Input: dimensioned drawing with shaded views. Units: mm. Origin: part minimum x, y, z. Give positions to 0.01 mm unless a question says otherwise; leave off trailing zeros. Write each loop counter-clockwise with the first axis right and the second up, starting at its lowest first coordinate (ties: lowest second). Pieces come first, ordered by that corner, then holes.
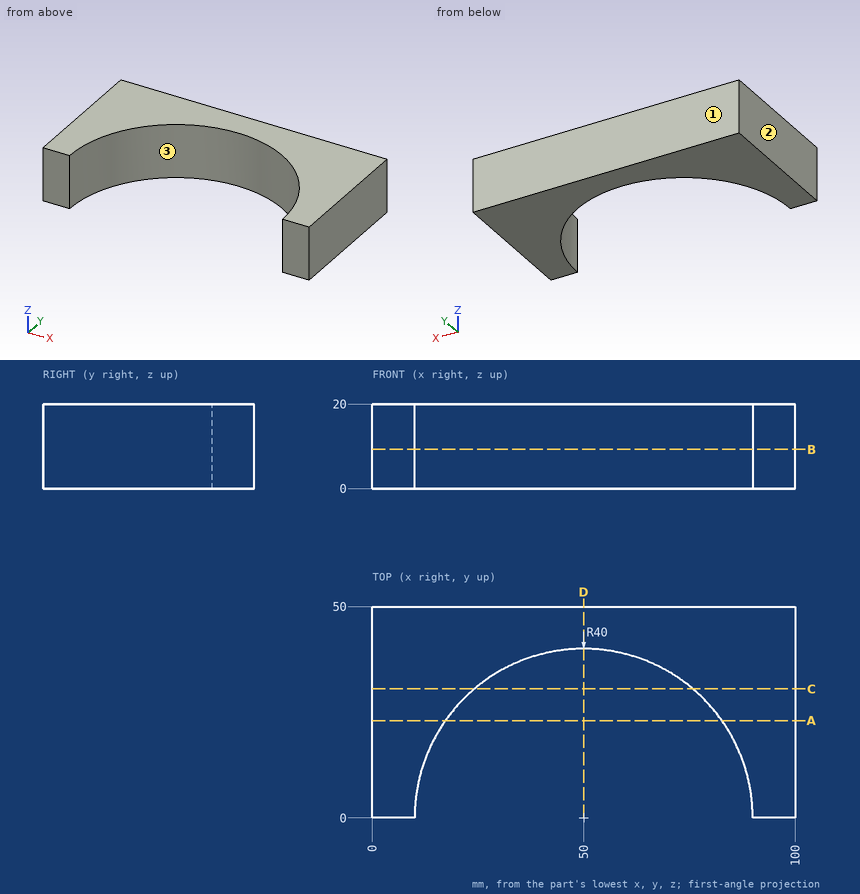
1. Line query: L1, parallel to Y at x = 50, z = 9; L2, parallel to X at y = 29, z = 17; L3, parallel to X at y = 19.5, z = 5.75. Output: solid intervals per line, ascending.
2. Mould query, pull axis X, two halves, no side actions, for the marked faces 1, 2 and 3. Classes: +X half, -X half, draft (parallel to the pull), parting line (faces both ways), or undercut.
3. Cut plane D-D, the plane x = 50. Return the cut outline in (y, z).
4. Cut plane C-C, the plane y = 30.5. Return the cut outline in (x, z).
5. Contact query for flat-ended pins moving along their axis: P1, Ø8, axis at y = 28, z = 8.5, coming from the -X side; P2, Ø2, axis at x = 21, z = 5.5, coming from the -Y side; P3, Ø1, axis at x = 80.5, z = 17.5, coming from the -Y side. Output: stop coordinate, or through.
6. Cut plane A-A, the plane y = 23. Return the cut outline in (x, z).
7. Cut plane B-B, the plane z = 9.25. Return the cut outline in (x, y), then the cut area to 3 significant figures.
Response values:
1. L1: y = 40 to 50
1. L2: x = 0 to 22.45, 77.55 to 100
1. L3: x = 0 to 15.08, 84.92 to 100
2. face 1: draft
2. face 2: -X half
2. face 3: undercut
3. outline: (40, 0) - (50, 0) - (50, 20) - (40, 20) - close
4. outline: (0, 0) - (24.12, 0) - (24.12, 20) - (0, 20) - close; (75.88, 0) - (100, 0) - (100, 20) - (75.88, 20) - close
5. P1: stops at x = 0
5. P2: stops at y = 26.46
5. P3: stops at y = 25.28
6. outline: (0, 0) - (17.27, 0) - (17.27, 20) - (0, 20) - close; (82.73, 0) - (100, 0) - (100, 20) - (82.73, 20) - close
7. outline: (0, 0) - (10, 0) arc R40 cw to (90, 0) - (100, 0) - (100, 50) - (0, 50) - close
7. area: 2,490 mm2
